```python
from build123d import *

# Parameters (mm, degrees)
SKETCH1_R                       = 1.5
BOSS_EXTRUDE1_DEPTH             = 3
BOSS_EXTRUDE2_DEPTH             = 18
BOSS_EXTRUDE2_DIRECTION_2_REACH = 78.19


with BuildPart() as part:
    # Sketch1 → Boss-Extrude1 (new body)
    with BuildSketch(Plane.YZ):
        Polygon((-9.054273726, -23.394917756), (28.546051212, -23.394917756), (28.546051212, -13.394917756), (47.945726274, -13.394917756), (50.945726274, -13.394917756), (50.945726274, 44.105082244), (-62.054273726, 44.105082244), (-62.054273726, -38.894917756), (-9.054273726, -38.894917756), align=None)
        with Locations(Location((-57.054273726, -33.894917756, 0), (0, 0, 270))):
            Circle(SKETCH1_R, mode=Mode.SUBTRACT)
        with Locations(Location((-57.054273726, 39.105082244, 0), (0, 0, 270))):
            Circle(SKETCH1_R, mode=Mode.SUBTRACT)
        with Locations(Location((45.945726274, 39.105082244, 0), (0, 0, 270))):
            Circle(SKETCH1_R, mode=Mode.SUBTRACT)
    extrude(amount=BOSS_EXTRUDE1_DEPTH)

    # Sketch2 → Boss-Extrude2 (add)
    with BuildSketch(Plane(origin=(0, 0, 0), x_dir=(0, -1, 0), z_dir=(-1, 0, 0))):
        Polygon((9.054273726, -23.394917756), (9.054273726, -25.394917756), (-28.546051212, -25.394917756), (-28.546051212, -23.394917756), (-28.546051212, -13.394917756), (-47.545726274, -13.394917756), (-47.545726274, -11.394917756), (-26.545726274, -11.394917756), (-26.545726274, -23.394917756), align=None)
    extrude(amount=BOSS_EXTRUDE2_DEPTH)

    # Boss-Extrude2 direction 2: up to this face of the body (flat: up to its plane)
    boss_extrude2_direction_2_end = Plane(part.part.faces().sort_by_distance((3, -9.750873795, 6.972989725))[0])
    # Sketch2 → Boss-Extrude2 direction 2 (add, up to the picked face)
    with BuildSketch(Plane(origin=(0, 0, 0), x_dir=(0, -1, 0), z_dir=(-1, 0, 0)), mode=Mode.PRIVATE) as boss_extrude2_direction_2_sk1:
        Polygon((9.054273726, -23.394917756), (9.054273726, -25.394917756), (-28.546051212, -25.394917756), (-28.546051212, -23.394917756), (-28.546051212, -13.394917756), (-47.545726274, -13.394917756), (-47.545726274, -11.394917756), (-26.545726274, -11.394917756), (-26.545726274, -23.394917756), align=None)
    boss_extrude2_direction_2_tool1 = split(extrude(boss_extrude2_direction_2_sk1.sketch, amount=-BOSS_EXTRUDE2_DIRECTION_2_REACH, mode=Mode.PRIVATE), bisect_by=boss_extrude2_direction_2_end, keep=Keep.BOTH, mode=Mode.PRIVATE)
    add(boss_extrude2_direction_2_tool1.solids().sort_by(Axis((0, -8.471216, -24.394918), (1, 0, 0)))[0])


solid = part.part
```
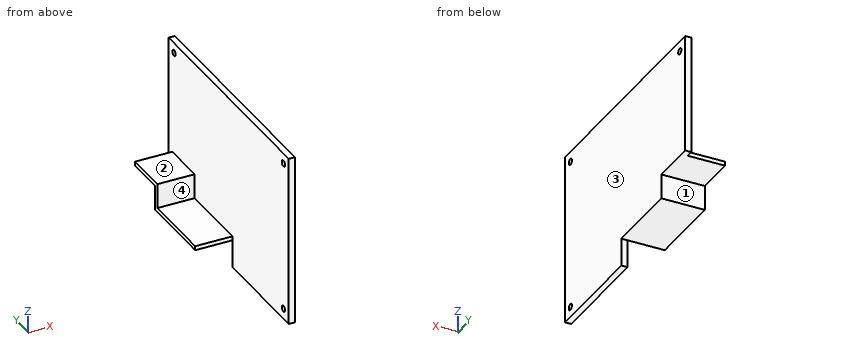
Can you work these out from the model? Positions are in its coordinate system, mm. Face numbers are marked on the shaded views. A direction names the side the tool comes from. Coordinates: 2 decimals unless noted, no trailing zeros. Loops run counter-clockwise (first coordinate to the right, second up) from the corner with the lowest first, then second, coordinate; pieces in that order, holes last. Notation, with made-up numbers: (-2.5, 16) -> (19.5, 16) arc R24 ccw to (19.5, 49) -> close; hole circle Ø10 at (20.25, -37.5). An arc over 180 degrees is marked (long way). Put each result on its own line as item: value. Start each with the question number.
Q1. I want a section at B-B (y = 23). Write out the boundary of the cut face in (x, z).
Q2. I want a section at A-A (x = -10). Write out the boundary of the cut face in (y, z), plus the area to 3 significant figures.
Q3. I'm going to push flat-ended pins straight in: P1, Ø4, axis at y = -57.05, z = -33.89, coming from the -X side; P2, Ø4, axis at x = -4, y = 23, coming from the -Z side; P3, Ø4, axis at x = -4, z = -21.5, coming from the -Y side; P4, Ø2.5, axis at y = -57.05, z = 39.11, coming from the -X side. Where does each tip first touch, or does it pass through?
Q4. I want a section at C-C (z = 0.5). Write out the boundary of the cut face in (x, y), plus the area to 3 significant figures.
Q5. For the marked faces 1, 2, 3 and 4, which set-ups out of +Z, -Z, +X, -X, +Y, -Y let a thin tool reach every point of the face, with its end or its side?
Q6. I want a section at D-D (y = -32.5). Write out the boundary of the cut face in (x, z), plus the area to 3 significant figures.
Q7. If I drill on line 1 (Y direction, x = 1.5, z = -34); line 2 (Z direction, x = -8, y = -3); line 3 (Z direction, x = -4.75, y = 36), over which ranges is the centre line in solid material (lowest first)? Write a range as [from, to].
Taken from the geometry:
1. outline: (-18, -25.39) -> (3, -25.39) -> (3, 44.11) -> (0, 44.11) -> (0, -23.39) -> (-18, -23.39) -> close
2. outline: (-9.05, -25.39) -> (28.55, -25.39) -> (28.55, -13.39) -> (47.55, -13.39) -> (47.55, -11.39) -> (26.55, -11.39) -> (26.55, -23.39) -> (-9.05, -23.39) -> close
2. area: 137 mm2
3. P1: stops at x = 0
3. P2: stops at z = -25.39
3. P3: stops at y = -9.05
3. P4: passes through
4. outline: (0, -62.05) -> (3, -62.05) -> (3, 50.95) -> (0, 50.95) -> close
4. area: 339 mm2
5. face 1: -Z, +X, -X, +Y
5. face 2: +Z, -X, +Y, -Y
5. face 3: +Z, -Z, +X, +Y, -Y
5. face 4: +Z, -X, -Y
6. outline: (0, -38.89) -> (3, -38.89) -> (3, 44.11) -> (0, 44.11) -> close
6. area: 249 mm2
7. line 1: y = [-62.05, -58.55], [-55.56, -9.05]
7. line 2: z = [-25.39, -23.39]
7. line 3: z = [-13.39, -11.39]
